For this review, take the finished solid that the model builds, in its own axes (mm). Face numbers are marked on the shaded views. A direction names the side the tool comes from. Round coordinates to 2 decimals unless told otherwise and drop trailing zeros. Order: outer loops, then holes, each group sorted by start corner. A loop starts at its lowest first (then second) coordinate and runs counter-clockwise, first axis right, second up. Notation, with made-up numbers: (24, 17.25) -> (55, 17.25) arc R6 ccw to (55, 25.25) -> close; hole circle Ø9 at (85, 35.25). An arc over 180 degrees is marked (long way). Use a Markdown table: item, result. Add a question column.
1) Machinability: for the marked faces 5 and 6, which of the approach directions +Z, -Z, +X, -X, +Y, -Y give a long, thin tool a straight path to every point of the face, cutting with its end or side? Answer none if there is none.
2) Consider section C-C (y = 2). State the section outline as (x, z) points, plus the area to 3 significant figures.
3) Wall thickness on line 1 along Z through (x, y) = (7.75, 3); line 2 along X through (y, z) = (0.6, -5); line 3 along Z through (x, y) = (-6, 3.25): over which ranges is each line inside the solid? List them lowest first. Write a range as [from, to].
4) Consider section B-B (z = -5). State the section outline as (x, y) points.
5) Consider section D-D (x = -7.5). Give the number of separate pieces and of enclosed holes in the cut face, plus the area to 3 significant figures.
6) Clearance check with flat-ended pins moving along their axes: P1, Ø3, axis at x = 7.5, z = -5.5, coming from the +Y side; P2, Ø10, axis at x = 1, z = -11.5, coming from the -Y side; P3, Ø13, axis at x = 0, z = -35, coming from the +Y side. State where each tip first meets the part, or that it passes through.
7) Draft analysis for pull direction X (two halves, no side actions). For the marked faces 1, 2, 3 and 4, state which applies: pulls with the +X half, pulls with the -X half, needs draft (parallel to the pull), parting line crosses it, or undercut.
8) Consider section A-A (x = 0). State the section outline as (y, z) points.
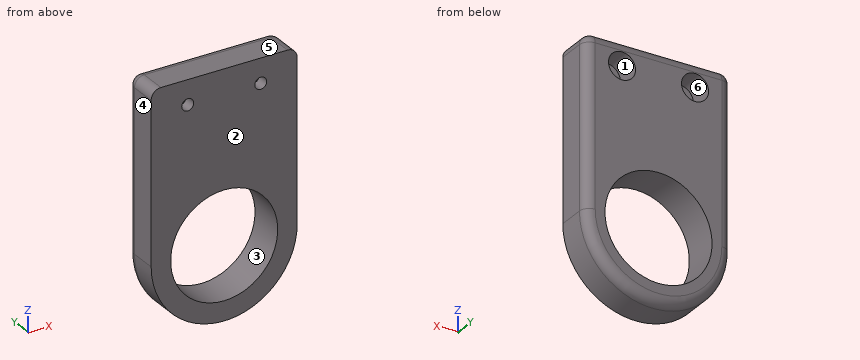
```python
from build123d import *

# Parameters (mm, degrees)
SKETCH1_R                                           = 11
BOSS_EXTRUDE1_DEPTH                                 = 7.5
CBORE_FOR_2_BINDING_HEAD_MACHINE_SCREW1_D           = 2.4384
CBORE_FOR_2_BINDING_HEAD_MACHINE_SCREW1_DEPTH       = 10
CBORE_FOR_2_BINDING_HEAD_MACHINE_SCREW1_CBORE_D     = 5.55752
CBORE_FOR_2_BINDING_HEAD_MACHINE_SCREW1_CBORE_DEPTH = 4.999999906
CBORE_FOR_2_BINDING_HEAD_MACHINE_SCREW1_TIP         = 0.732569267
FILLET1_R                                           = 2


with BuildPart() as part:
    # Sketch1 → Boss-Extrude1 (new body)
    with BuildSketch(Plane(origin=(0, 0, 0), x_dir=(1, 0, 0), z_dir=(0, 1, 0))):
        with BuildLine():
            Line((-15, 0), (15, 0))
            Line((15, 0), (15, 35))
            ThreePointArc((15, 35), (0, 50), (-15, 35))
            Line((-15, 35), (-15, 0))
        make_face()
        with Locations(Location((0, 35, 0), (0, 0, 270))):
            Circle(SKETCH1_R, mode=Mode.SUBTRACT)
    extrude(amount=BOSS_EXTRUDE1_DEPTH)

    # CBORE for #2 Binding Head Machine Screw1
    with Locations(Plane(origin=(0, 7.5, 0), x_dir=(1, 0, 0), z_dir=(0, 1, 0))):
        with Locations((-7.5, 5), (7.5, 5)):
            CounterBoreHole(CBORE_FOR_2_BINDING_HEAD_MACHINE_SCREW1_D / 2, CBORE_FOR_2_BINDING_HEAD_MACHINE_SCREW1_CBORE_D / 2, CBORE_FOR_2_BINDING_HEAD_MACHINE_SCREW1_CBORE_DEPTH, depth=CBORE_FOR_2_BINDING_HEAD_MACHINE_SCREW1_DEPTH)
            with Locations((0, 0, -(CBORE_FOR_2_BINDING_HEAD_MACHINE_SCREW1_DEPTH + CBORE_FOR_2_BINDING_HEAD_MACHINE_SCREW1_TIP / 2))):  # 118° drill point
                Cone(0, CBORE_FOR_2_BINDING_HEAD_MACHINE_SCREW1_D / 2, CBORE_FOR_2_BINDING_HEAD_MACHINE_SCREW1_TIP, mode=Mode.SUBTRACT)

    # Fillet1
    fillet1_edges = [part.edges().sort_by_distance(p)[0] for p in [
        (15, 7.5, -17.5),
        (0, 7.5, -50),
        (-15, 7.5, -17.5),
        (15, 3.75, 0),
        (-15, 3.75, 0),
        (0, 7.5, 0),
    ]]
    fillet(fillet1_edges, radius=FILLET1_R)


solid = part.part
```
Results list:
| question | item | result |
|---|---|---|
| 1 | face 5 | +Z, +X, -X, +Y, -Y |
| 1 | face 6 | +Y |
| 2 | outline | (-15, -35) arc R15 ccw to (15, -35) -> (15, -2) arc R2 ccw to (13, 0) -> (-13, 0) arc R2 ccw to (-15, -2) -> close; hole circle Ø22 at (0, -35); hole circle Ø2.44 at (-7.5, -5); hole circle Ø2.44 at (7.5, -5) |
| 2 | area | 1,010 mm2 |
| 3 | line 1 | [-47.84, -42.81], [-27.19, -7.77], [-2.23, 0] |
| 3 | line 2 | [-15, -8.72], [-6.28, 6.28], [8.72, 15] |
| 3 | line 3 | [-48.75, -44.22], [-25.78, -7.34], [-2.66, 0] |
| 4 | outline | (-15, 0) -> (-8.72, 0) -> (-8.72, 2.5) -> (-10.28, 2.5) -> (-10.28, 7.5) -> (-13, 7.5) arc R2 ccw to (-15, 5.5) -> close; (-6.28, 0) -> (6.28, 0) -> (6.28, 2.5) -> (4.72, 2.5) -> (4.72, 7.5) -> (-4.72, 7.5) -> (-4.72, 2.5) -> (-6.28, 2.5) -> close; (8.72, 0) -> (15, 0) -> (15, 5.5) arc R2 ccw to (13, 7.5) -> (10.28, 7.5) -> (10.28, 2.5) -> (8.72, 2.5) -> close |
| 5 | separate pieces | 3 |
| 5 | enclosed holes | 0 |
| 5 | area | 203 mm2 |
| 6 | P1 | y = 2.5 |
| 6 | P2 | y = 0 |
| 6 | P3 | through |
| 7 | face 1 | undercut |
| 7 | face 2 | needs draft |
| 7 | face 3 | undercut |
| 7 | face 4 | pulls with the -X half |
| 8 | outline | (0, -50) -> (5.5, -50) arc R2 ccw to (7.5, -48) -> (7.5, -46) -> (0, -46) -> close; (0, -24) -> (7.5, -24) -> (7.5, -2) arc R2 ccw to (5.5, 0) -> (0, 0) -> close |
